Design review of the part built by this model. Coordinates are the model's own, in mm. Face numbers are marked on the shaded views. A direction names the side the tool comes from. Round coordinates to 2 decimals unless told otherwise and drop trailing zeros. Write each loop counter-clockwise with the first axis right and the second up, starting at its lowest first coordinate (ties: lowest second). Pieces come first, ordered by that corner, then holes. Notation, with made-up numbers: M 0.5,44 L 32.5,44 A12 cw 32.5,53 Z; hole C -10.5,-9 d2. An arc over 180 degrees is marked long. One line per question, with ' | ' between items. Start each with the question number.
Item 1: Draft analysis for pull direction Z (two halves, no side actions). For the marked faces 1 and 2, state which applies: released by +Z, released by -Z, zero draft, split by the parting line, or undercut.
Item 2: For L1, parallel to X at y = 7.75, z = 0; L2, parallel to X at y = -2.5, z = 31; L3, parallel to Y at x = 75, z = 40, list the stretches that pass through material, from the lowest coordinate up.
Item 3: Add section C-C, the plane x = -9. State the section outline as (y, z) points, and give its area (3 significant figures).
Item 4: Add section D-D, the plane z = 0. State the section outline as (x, y) points.
Item 5: Insertion check: pin 1 Ø6 at (x, z) = (79.5, 31.5) entering from +Y; pin 2 Ø8 at (x, z) = (-35, -43.5) entering from +Y; pin 3 Ø1 at (x, y) = (-61, 2.5) entering from +Z; pin 4 Ø3 at (x, y) = (-42, 5.5) entering from -Z. Each pin has a flat end and moves straight along its axis. Give the tip position at first contact, or say it passes through.
Item 6: Add section B-B, the plane y = 7.75. State the section outline as (x, z) points, and give its area (3 significant figures).
Item 7: Add section A-A, the plane z = -31.5. State the section outline as (x, y) points, and give its area (3 significant figures).
Item 8: Machinability: for the marked faces 3 and 4, which of the approach directions +Z, -Z, +X, -X, +Y, -Y give a long, thin tool a straight path to every point of the face, cutting with its end or side? Answer none if there is none.
```python
from build123d import *

# Parameters (mm, degrees)
SKETCH1_W           = 174
SKETCH1_H           = 78
SKETCH1_R           = 2.5
SKETCH1_R_2         = 34
BOSS_EXTRUDE1_DEPTH = 10
BOSS_EXTRUDE2_START = -5
SKETCH1_3_W         = 174
SKETCH1_3_H         = 78
SKETCH1_3_R         = 2.5
SKETCH1_3_R_2       = 34
SKETCH1_3_H_2       = 10
BOSS_EXTRUDE2_DEPTH = 5


with BuildPart() as part:
    # Sketch1 → Boss-Extrude1 (new body)
    with BuildSketch(Plane(origin=(0, 0, 0), x_dir=(1, 0, 0), z_dir=(0, 1, 0))):
        Rectangle(SKETCH1_W, SKETCH1_H)
        with Locations(Location((79.5, 31.5, 0), (0, 0, 270))):
            Circle(SKETCH1_R, mode=Mode.SUBTRACT)
        with Locations(Location((79.5, -31.5, 0), (0, 0, 270))):
            Circle(SKETCH1_R, mode=Mode.SUBTRACT)
        with Locations(Location((-79.5, -31.5, 0), (0, 0, 270))):
            Circle(SKETCH1_R, mode=Mode.SUBTRACT)
        with Locations(Location((-79.5, 31.5, 0), (0, 0, 270))):
            Circle(SKETCH1_R, mode=Mode.SUBTRACT)
        with Locations(Location((-48, 0, 0), (0, 0, 270))):
            Circle(SKETCH1_R_2, mode=Mode.SUBTRACT)
        with Locations(Location((48, 0, 0), (0, 0, 270))):
            Circle(SKETCH1_R_2, mode=Mode.SUBTRACT)
    extrude(amount=BOSS_EXTRUDE1_DEPTH)

    # Sketch1_3 → Boss-Extrude2 (add)
    # profile 1 of 5: a face of its own
    with BuildSketch(Plane(origin=(0, 0, 0), x_dir=(1, 0, 0), z_dir=(0, 1, 0)).offset(BOSS_EXTRUDE2_START)):
        Rectangle(SKETCH1_3_W, SKETCH1_3_H)
        with Locations(Location((79.5, 31.5, 0), (0, 0, 270))):
            Circle(SKETCH1_3_R, mode=Mode.SUBTRACT)
        with Locations(Location((79.5, -31.5, 0), (0, 0, 270))):
            Circle(SKETCH1_3_R, mode=Mode.SUBTRACT)
        with Locations(Location((-79.5, -31.5, 0), (0, 0, 270))):
            Circle(SKETCH1_3_R, mode=Mode.SUBTRACT)
        with Locations(Location((-79.5, 31.5, 0), (0, 0, 270))):
            Circle(SKETCH1_3_R, mode=Mode.SUBTRACT)
        with Locations(Location((-48, 0, 0), (0, 0, 270))):
            Circle(SKETCH1_3_R_2, mode=Mode.SUBTRACT)
        with Locations(Location((48, 0, 0), (0, 0, 270))):
            Circle(SKETCH1_3_R_2, mode=Mode.SUBTRACT)
    # profile 2 of 5: a face of its own
    with BuildSketch(Plane(origin=(0, 0, 0), x_dir=(1, 0, 0), z_dir=(0, 1, 0)).offset(BOSS_EXTRUDE2_START)):
        with Locations(Location((48, 0, 0), (0, 0, 270))):
            Circle(SKETCH1_3_R_2)
    # profile 3 of 5: a face of its own
    with BuildSketch(Plane(origin=(0, 0, 0), x_dir=(1, 0, 0), z_dir=(0, 1, 0)).offset(BOSS_EXTRUDE2_START)):
        with Locations((0, -44)):
            Rectangle(SKETCH1_3_W, SKETCH1_3_H_2)
    # profile 4 of 5: a face of its own
    with BuildSketch(Plane(origin=(0, 0, 0), x_dir=(1, 0, 0), z_dir=(0, 1, 0)).offset(BOSS_EXTRUDE2_START)):
        with Locations((0, 44)):
            Rectangle(SKETCH1_3_W, SKETCH1_3_H_2)
    # profile 5 of 5: a face of its own
    with BuildSketch(Plane(origin=(0, 0, 0), x_dir=(1, 0, 0), z_dir=(0, 1, 0)).offset(BOSS_EXTRUDE2_START)):
        with Locations(Location((-48, 0, 0), (0, 0, 270))):
            Circle(SKETCH1_3_R_2)
    extrude(amount=BOSS_EXTRUDE2_DEPTH)


solid = part.part
```
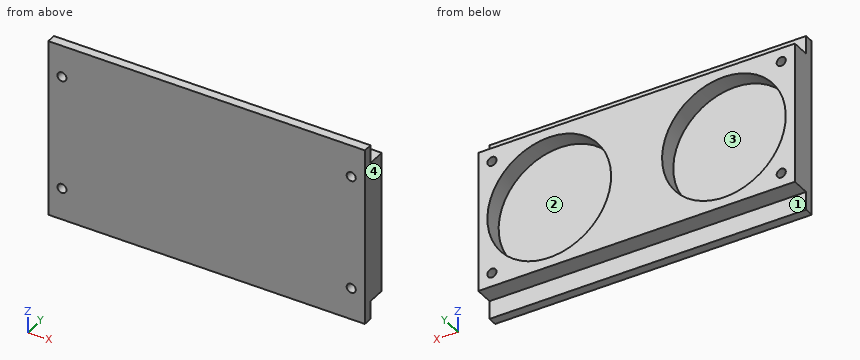
Computed values:
1) face 1: zero draft | face 2: undercut
2) L1: x = -87 to -82, -14 to 14, 82 to 87 | L2: x = -87 to -81.95, -77.05 to 77.05, 81.95 to 87 | L3: y = -5 to 0
3) outline: M -5,-49 L 0,-49 L 0,-39 L 10,-39 L 10,39 L 0,39 L 0,49 L -5,49 Z | area: 1,270 mm^2
4) outline: M -87,-5 L 87,-5 L 87,10 L 82,10 L 82,0 L 14,0 L 14,10 L -14,10 L -14,0 L -82,0 L -82,10 L -87,10 Z
5) pin 1: stops at y = 10 | pin 2: stops at y = 0 | pin 3: stops at z = 39 | pin 4: stops at z = -39
6) outline: M -87,-39 L 87,-39 L 87,39 L -87,39 Z; hole C -79.5,-31.5 d5; hole C -48,0 d68; hole C -79.5,31.5 d5; hole C 48,0 d68; hole C 79.5,-31.5 d5; hole C 79.5,31.5 d5 | area: 6,230 mm^2
7) outline: M -87,-5 L -82,-5 L -82,10 L -87,10 Z; M -77,-5 L 77,-5 L 77,10 L 60.8,10 L 60.8,0 L 35.2,0 L 35.2,10 L -35.2,10 L -35.2,0 L -60.8,0 L -60.8,10 L -77,10 Z; M 82,-5 L 87,-5 L 87,10 L 82,10 Z | area: 1,950 mm^2
8) face 3: +Y | face 4: +Z, -Z, +X, +Y, -Y
